Source: CAD feature listing. Evaluate the final solid. Frame: model axes, mm. A direction names the side the tool comes from. Give positions to 0.01 mm unless a question says otherwise; leave off trailing zeros. Order: outer loops, then holes, each group sorted by start corner. A loop starts at its lowest first (then second) coordinate and runs counter-clockwise, first axis right, second up. Notation, with made-up numbers: (52, 53.5) -> (90, 53.5) arc R29 ccw to (90, 77.5) -> close; hole circle Ø3 at (10.5, -1). An arc over 180 degrees is marked (long way). Answer in a Markdown table with one row per item.
```python
from build123d import *

# Parameters (mm, degrees)
CROQUIS1_W              = 26
CROQUIS1_H              = 27
SALIENTE_EXTRUIR1_DEPTH = 2
CROQUIS2_W              = 26
CROQUIS2_H              = 1
SALIENTE_EXTRUIR2_DEPTH = 13
SALIENTE_EXTRUIR3_DEPTH = 9
CROQUIS5_R              = 2.7
CORTAR_EXTRUIR1_DEPTH   = 17
REDONDEO1_R             = 3
CORTAR_EXTRUIR2_START   = -27
CORTAR_EXTRUIR2_DEPTH   = 27


with BuildPart() as part:
    # Croquis1 → Saliente-Extruir1 (new body)
    with BuildSketch(Plane.XY):
        with Locations((-26.399771714, -2.880068531)):
            Rectangle(CROQUIS1_W, CROQUIS1_H)
    extrude(amount=SALIENTE_EXTRUIR1_DEPTH)

    # Croquis2 → Saliente-Extruir2 (add)
    with BuildSketch(Plane.XY.offset(2)):
        with Locations((-26.399771714, 10.119931469)):
            Rectangle(CROQUIS2_W, CROQUIS2_H)
        with Locations((-26.399771714, -15.880068531)):
            Rectangle(CROQUIS2_W, CROQUIS2_H)
    extrude(amount=SALIENTE_EXTRUIR2_DEPTH)

    # Croquis3 → Saliente-Extruir3 (add)
    with BuildSketch(Plane(origin=(-13.399771714, 0, 0), x_dir=(0, 0, -1), z_dir=(1, 0, 0))):
        Polygon((-17, -16.380068531), (-15, -15.380068531), (-15, -16.380068531), (-13, -16.380068531), (-13, -22.880068531), (-15, -22.880068531), (-17, -22.880068531), align=None)
        Polygon((-15, 10.619931469), (-13, 10.619931469), (-13, 17.119931469), (-15, 17.119931469), (-17, 17.119931469), (-17, 10.619931469), (-15, 9.619931469), align=None)
    extrude(amount=-SALIENTE_EXTRUIR3_DEPTH)

    # Croquis5 → Cortar-Extruir1 (cut)
    with BuildSketch(Plane.XY.offset(17)):
        with Locations(Location((-17.899771714, -18.880068531, 0), (0, 0, 67.808393434))):
            Circle(CROQUIS5_R)
        with Locations(Location((-17.899771714, 13.119931469, 0), (0, 0, 292.191606566))):
            Circle(CROQUIS5_R)
    extrude(amount=-CORTAR_EXTRUIR1_DEPTH, mode=Mode.SUBTRACT)

    # Redondeo1
    redondeo1_edges = [part.edges().sort_by_distance(p)[0] for p in [
        (-22.399771714, -22.880068531, 15),
        (-13.399771714, -22.880068531, 15),
        (-22.399771714, 17.119931469, 15),
        (-13.399771714, 17.119931469, 15),
    ]]
    fillet(redondeo1_edges, radius=REDONDEO1_R)

    # Croquis6 → Cortar-Extruir2 (cut)
    with BuildSketch(Plane.XZ.offset(16.380068531).offset(CORTAR_EXTRUIR2_START)):
        Polygon((-39.399771714, 15), (-39.399771714, 8), (-32.399771714, 15), align=None)
    extrude(amount=CORTAR_EXTRUIR2_DEPTH, mode=Mode.SUBTRACT)


solid = part.part
```
(1) First-contact query: pin 1 Ø3 at (x, z) = (-14.5, 6.5) entering from -Y; pin 2 Ø6 at (y, z) = (-17.5, 11) entering from -X; pin 3 Ø2 at (y, z) = (11, 15.5) entering from -X; pin 4 Ø2 at (y, z) = (12.5, 8) entering from +X. Flat tips, straight axial feed; report the tip coordinate or a pass-through.
A:
| item | result |
|---|---|
| pin 1 | stops at y = -16.38 |
| pin 2 | stops at x = -39.18 |
| pin 3 | stops at x = -32.82 |
| pin 4 | passes through |
(2) Section query A-A (z = 3.25). Return the cut outline in (x, y), plus the area to 3 significant figures.
A:
| item | result |
|---|---|
| outline | (-39.4, -16.38) -> (-18.92, -16.38) arc R2.7 cw to (-16.88, -16.38) -> (-13.4, -16.38) -> (-13.4, -15.38) -> (-39.4, -15.38) -> close; (-39.4, 9.62) -> (-13.4, 9.62) -> (-13.4, 10.62) -> (-16.88, 10.62) arc R2.7 cw to (-18.92, 10.62) -> (-39.4, 10.62) -> close |
| area | 51.5 mm^2 |
(3) Ray query, probe 1 along Y at (x, z) = (-21.75, 10); probe 2 along Y at (x, z) = (-17, 14.5); probe 3 along Z at (x, y) = (-29.5, 7). Return the intervals inside material, ascending.
A:
| item | result |
|---|---|
| probe 1 | y = -16.38 to -15.38, 9.62 to 10.62 |
| probe 2 | y = -22.88 to -21.43, -16.33 to -15.38, 9.62 to 10.57, 15.67 to 17.12 |
| probe 3 | z = 0 to 2 |
(4) Section query B-B (z = 13.5). Return the cut outline in (x, y), plus the area to 3 significant figures.
A:
| item | result |
|---|---|
| outline | (-33.9, -16.38) -> (-22.4, -16.38) -> (-22.4, -19.88) arc R3 ccw to (-19.4, -22.88) -> (-16.4, -22.88) arc R3 ccw to (-13.4, -19.88) -> (-13.4, -15.38) -> (-33.9, -15.38) -> close; (-33.9, 9.62) -> (-13.4, 9.62) -> (-13.4, 14.12) arc R3 ccw to (-16.4, 17.12) -> (-19.4, 17.12) arc R3 ccw to (-22.4, 14.12) -> (-22.4, 10.62) -> (-33.9, 10.62) -> close; hole circle Ø5.4 at (-17.9, -18.88); hole circle Ø5.4 at (-17.9, 13.12) |
| area | 104 mm^2 |
(5) Pull-direction query (Y, two-part tool) for faces 5 (the cylindrical face through (-21.54, -21.98, 14.97)), 6 (the flat face through (-17.837, -15.887, 16.014)), 7 (the flat face through (-22.4, -18, 15)); classes: +Y half, -Y half, draft (parallel to the pull), parting line (faces both ways), or undercut.
A:
| item | result |
|---|---|
| face 5 | -Y half |
| face 6 | undercut |
| face 7 | draft |
(6) Section query D-D (x = -36). Return the cut outline in (y, z).
A:
| item | result |
|---|---|
| outline | (-16.38, 0) -> (10.62, 0) -> (10.62, 11.4) -> (9.62, 11.4) -> (9.62, 2) -> (-15.38, 2) -> (-15.38, 11.4) -> (-16.38, 11.4) -> close |
(7) Section query C-C (y = -18). Return the cut outline in (x, z), plus the area to 3 significant figures.
A:
| item | result |
|---|---|
| outline | (-22.4, 13) -> (-20.45, 13) -> (-20.45, 17) -> (-22.4, 17) -> close; (-15.35, 13) -> (-13.4, 13) -> (-13.4, 17) -> (-15.35, 17) -> close |
| area | 15.6 mm^2 |
(8) Access query for faces 1 (the flat face through (-18, 16, 13)), 2 (the flat face through (-27, -3, 2)), 3 (the flat face through (-15, -16.38, 6)), 4 (the flat face through (-27, -16, 15)). Directions: +Z, -Z, +X, -X, +Y, -Y. A direction counts if a zero-diameter tool reaches every point of the face in a straight line with its end or side. Return the directions, or none.
A:
| item | result |
|---|---|
| face 1 | -Z, +X, -X, +Y |
| face 2 | +Z, +X, -X |
| face 3 | -Z, +X, -X, -Y |
| face 4 | +Z, -X, +Y, -Y |
